```python
from build123d import *

# Parameters (mm, degrees)
SKETCH_W           = 3
SKETCH_H           = 15
PAD_DEPTH          = 15
THICKNESS_T        = 1
THICKNESS_FACE2_W  = 3
THICKNESS_FACE2_H  = 15
POCKET_DEPTH       = 5
POCKET_FACE4_W     = 15
POCKET_FACE4_H     = 3
POCKET001_DEPTH    = 5
POCKET001_FACE18_W = 3
POCKET001_FACE18_H = 1
POCKET002_DEPTH    = 5
PAD001_DEPTH       = 10


with BuildPart() as part:
    # Sketch → Pad (new body)
    with BuildSketch(Plane.XY):
        with Locations((1.5, 7.5)):
            Rectangle(SKETCH_W, SKETCH_H)
    extrude(amount=PAD_DEPTH)

    # Thickness
    thickness_openings = [part.faces().sort_by_distance(p)[0] for p in [
        (1.5, 0, 7.5),
    ]]
    offset(amount=THICKNESS_T, openings=thickness_openings)

    # Thickness Face2 → Pocket (cut)
    with BuildSketch(Plane(origin=(1.5, 15, 7.5), x_dir=(-1, 0, 0), z_dir=(0, -1, 0))):
        Rectangle(THICKNESS_FACE2_W, THICKNESS_FACE2_H)
    extrude(amount=-POCKET_DEPTH, mode=Mode.SUBTRACT)

    # Pocket Face4 → Pocket001 (cut)
    with BuildSketch(Plane(origin=(1.5, 7.5, 0), x_dir=(0, 1, 0), z_dir=(0, 0, 1))):
        Rectangle(POCKET_FACE4_W, POCKET_FACE4_H)
    extrude(amount=-POCKET001_DEPTH, mode=Mode.SUBTRACT)

    # Pocket001 Face18 → Pocket002 (cut)
    with BuildSketch(Plane(origin=(1.5, 15, -0.5), x_dir=(-1, 0, 0), z_dir=(0, -1, 0))):
        Rectangle(POCKET001_FACE18_W, POCKET001_FACE18_H)
    extrude(amount=-POCKET002_DEPTH, mode=Mode.SUBTRACT)

    # Pocket002 Face2 → Pad001 (add)
    with BuildSketch(Plane(origin=(1.5, 0, 8.164055), x_dir=(-1, 0, 0), z_dir=(0, -1, 0))):
        with BuildLine():
            Line((1.5, 8.164055), (1.5, -6.835945))
            Line((1.5, -6.835945), (-1.5, -6.835945))
            Line((-1.5, -6.835945), (-1.5, 8.164055))
            Line((-1.5, 8.164055), (-1.5, 9.164055))
            ThreePointArc((-1.5, 9.164055), (-2.207107, 8.871162), (-2.5, 8.164055))
            Line((-2.5, 8.164055), (-2.5, -6.835945))
            ThreePointArc((-2.5, -6.835945), (-2.207107, -7.543052), (-1.5, -7.835945))
            Line((-1.5, -7.835945), (1.5, -7.835945))
            ThreePointArc((1.5, -7.835945), (2.207107, -7.543052), (2.5, -6.835945))
            Line((2.5, -6.835945), (2.5, 8.164055))
            ThreePointArc((2.5, 8.164055), (2.207107, 8.871162), (1.5, 9.164055))
            Line((1.5, 9.164055), (1.5, 8.164055))
        make_face()
    extrude(amount=PAD001_DEPTH)


solid = part.part
```
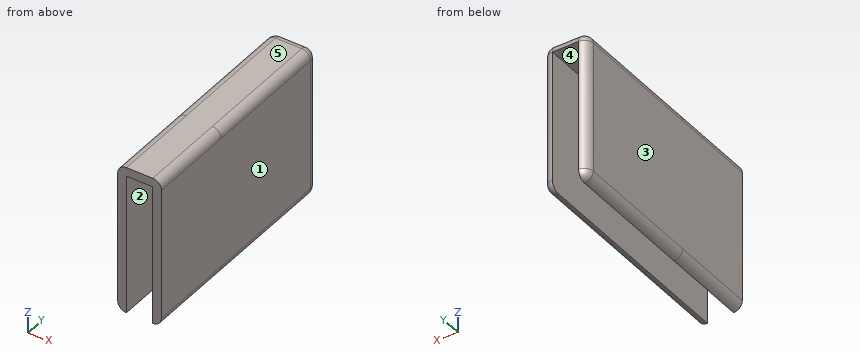
Geometry check sheet. Reference: the model listing, model coordinates, mm. Face numbers are marked on the shaded views. A direction names the side the tool comes from. Round coordinates to 2 decimals unless told otherwise and drop trailing zeros. Write each loop counter-clockwise with the first axis right and the second up, starting at its lowest first coordinate (ties: lowest second). Pieces come first, ordered by that corner, then holes. Notation, with made-up numbers: (-26.5, 25.25) -> (20.5, 25.25) arc R18 cw to (20.5, 45.25) -> close; hole circle Ø9 at (78.25, 51). An arc over 180 degrees is marked (long way). Put each result on its own line as item: value.
1) Release check for a two-part mould opening along X. For the marked faces 3, 4 and 5 record: pulls with the +X half, pulls with the -X half, needs draft (parallel to the pull), parting line crosses it, or undercut.
Recorded:
face 3: pulls with the -X half
face 4: undercut
face 5: needs draft
2) Access from +Z, -Z, +X, -X, +Y, -Y to the whole of each face (thin tool, end or side, straight path). Record for the marked faces 1 and 2.
Recorded:
face 1: +Z, -Z, +X, +Y, -Y
face 2: -Z, +Y, -Y
3) Cross-section at D-D, the plane x = 0.7. Enter the section's corners in (y, z), plus the area to 3 significant figures.
Recorded:
outline: (-10, 15) -> (16, 15) arc R1 ccw to (15, 16) -> (-10, 16) -> close
area: 25.8 mm2
4) Thickness scan on probe 1 along X at (y, z) = (7.25, 7.5); probe 2 along Z at (x, y) = (2.8, -5.25); probe 3 along Z at (x, y) = (-0.15, 5.5). Record the ranges inside material, lowest first. Write a range as from..to.
Recorded:
probe 1: x = -1..0, 3..4
probe 2: z = 15..16
probe 3: z = -0.99..15.99
5) Cross-section at C-C, the plane x = -0.65. Enter the section's corners in (y, z).
Recorded:
outline: (-10, -0.76) -> (15, -0.76) arc R0.76 ccw to (15.76, 0) -> (15.76, 15) arc R0.76 ccw to (15, 15.76) -> (-10, 15.76) -> close
6) Cross-section at A-A, the plane z = 1.5. Enter the section's corners in (x, y).
Recorded:
outline: (-1, -10) -> (0, -10) -> (0, 16) arc R1 ccw to (-1, 15) -> close; (3, -10) -> (4, -10) -> (4, 15) arc R1 ccw to (3, 16) -> close
7) Cross-section at B-B, the plane y = 13.5. Enter the section's corners in (x, z), plus the area to 3 significant figures.
Recorded:
outline: (-1, 0) arc R1 ccw to (0, -1) -> (0, 15) -> (3, 15) -> (3, -1) arc R1 ccw to (4, 0) -> (4, 15) arc R1 ccw to (3, 16) -> (0, 16) arc R1 ccw to (-1, 15) -> close
area: 36.1 mm2
8) Depth check by flat-ended pin: P1, Ø1.5, axis at x = 2, y = -2.5, coming from the -Z side. Enter the tip coordinate at first touch or a pass-through.
Recorded:
P1: stops at z = 15
